```python
from build123d import *

# Parameters (mm, degrees)
BOSS_EXTRUDE1_DEPTH = 6
SKETCH2_W           = 50
SKETCH2_H           = 25
SKETCH3_R           = 16
CUT_EXTRUDE1_DEPTH  = 198.288440507


with BuildPart() as part:
    # Sketch1 → Boss-Extrude1 (new, symmetric)
    with BuildSketch(Plane(origin=(0, 0, 0), x_dir=(0, 0, -1), z_dir=(1, 0, 0))):
        with BuildLine():
            Line((0, 167.5), (-8, 167.5))
            Line((-8, 167.5), (-8, 178.988731807))
            Line((-8, 178.988731807), (-48, 178.988731807))
            ThreePointArc((-48, 178.988731807), (-79.124980803, 0), (-48, -178.988731807))
            Line((-48, -178.988731807), (-8, -178.988731807))
            Line((-8, -178.988731807), (-8, -167.5))
            Line((-8, -167.5), (0, -167.5))
            Line((0, -167.5), (0, -127.5))
            Line((0, -127.5), (-11.889594458, -127.5))
            ThreePointArc((-11.889594458, -127.5), (-29.124980803, 0), (-11.889594458, 127.5))
            Line((-11.889594458, 127.5), (0, 127.5))
            Line((0, 127.5), (0, 167.5))
        make_face()
    extrude(amount=BOSS_EXTRUDE1_DEPTH, both=True)

    # Sketch2 → Revolve1 (revolve)
    with BuildSketch(Plane(origin=(0, 0, 0), x_dir=(0, 0, -1), z_dir=(1, 0, 0))):
        with Locations((-54.124980803, 12.5)):
            Rectangle(SKETCH2_W, SKETCH2_H)
    revolve(axis=Axis((0, 0, 29.124980803), (0, 0, 1)))

    # Sketch3 → Cut-Extrude1 (cut, through all)
    with BuildSketch(Plane.XY):
        with Locations(Location((0, 0, 0), (0, 0, 247.975687163))):
            Circle(SKETCH3_R)
    extrude(amount=CUT_EXTRUDE1_DEPTH, mode=Mode.SUBTRACT)


solid = part.part
```
CAD build for the part. Positions are in the model's coordinates, mm. A direction names the side the tool comes from. Round coordinates to 2 decimals unless told otherwise and drop trailing zeros. Loops run counter-clockwise (first coordinate to the right, second up) from the corner with the lowest first, then second, coordinate; pieces in that order, holes last. Notation, with made-up numbers: M -37,81.5 L 4,81.5 A13 ccw 4,97.5 Z; hole C 17.5,-15.5 d6. An arc over 180 degrees is marked long. Use a Markdown table: item, result. Add a question column.
(1) Which spindle directions (+Z, -Z, +X, -X, +Y, -Y) get a long thin tool onto all of the face, cutting with end or side? Do faces 1 (the face through (-18, 0, 29.125)), 2 (the face through (0, 127.5, 6)), 3 (the face through (0, 167.5, 4)), 4 (the face through (0, -173, 8)), 5 (the face through (6, -114, 40)). Say none if no direction does.
(2) Cut at C-C (z = 15.5). Give the cut face in (x, y).
(3) Flat gauge pins, fed straight in: pin 1 (9.5 mm diameter, centred on x = 19, y = 9.5, fed in from -Z) (3 decimals); pin 2 (6.5 mm diameter, centred on x = 0.5, z = 3.5, fed in from +Y); pin 3 (1 mm diameter, centred on y = -138, z = 30, fed in from +X). Where does each tip first touch, or does it go through?
(4) Cut at A-A (y = 0). Give the cut face in (x, z), and give its area (3 significant figures).
(5) Cut at B-B (x = 0). Give the cut face in (y, z), and give its area (3 significant figures).
(6) Cut at D-D (z = 53). Give the cut face in (x, y), and give its area (3 significant figures).
(7) Drill centre lines: line 1 (X direction, y = 0, z = 59); line 2 (X direction, y = 79, z = 50); line 3 (Y direction, x = 0.5, z = 36.5). Where is each one in solid material? Low to high.
Geometry says:
| question | item | result |
|---|---|---|
| 1 | face 1 | -Z, -X, +Y, -Y |
| 1 | face 2 | -Z, +X, -X |
| 1 | face 3 | -Z, +X, -X, +Y |
| 1 | face 4 | -Z, +X, -X, -Y |
| 1 | face 5 | +Z, -Z, +X, -Y |
| 2 | outline | M -6,-178.99 L 6,-178.99 L 6,-113.58 L -6,-113.58 Z; M -6,113.58 L 6,113.58 L 6,178.99 L -6,178.99 Z |
| 3 | pin 1 | stops at z = 29.125 |
| 3 | pin 2 | stops at y = 167.5 |
| 3 | pin 3 | stops at x = 6 |
| 4 | outline | M -25,29.12 L -16,29.12 L -16,79.12 L -25,79.12 Z; M 16,29.12 L 25,29.12 L 25,79.12 L 16,79.12 Z |
| 4 | area | 900 mm² |
| 5 | outline | M -178.99,8 L -167.5,8 L -167.5,0 L -127.5,0 L -127.5,11.89 A480.21 cw -16,28.86 L -16,79.12 L -25,79.12 L -25,78.54 A530.21 ccw -178.99,48 Z; M 16,28.86 A480.21 cw 127.5,11.89 L 127.5,0 L 167.5,0 L 167.5,8 L 178.99,8 L 178.99,48 A530.21 ccw 25,78.54 L 25,79.12 L 16,79.12 Z |
| 5 | area | 16,900 mm² |
| 6 | outline | M -6,-164.38 L 6,-164.38 L 6,-24.27 A25 ccw 6,24.27 L 6,164.38 L -6,164.38 L -6,24.27 A25 ccw -6,-24.27 Z; hole C 0,0 d32 |
| 6 | area | 4,510 mm² |
| 7 | line 1 | x = -25 to -16, 16 to 25 |
| 7 | line 2 | x = -6 to 6 |
| 7 | line 3 | y = -178.99 to -15.99, 15.99 to 178.99 |
